```python
from build123d import *

# Parameters (mm, degrees)
BOSS_EXTRU_2_DEPTH   = 5
D_GAGEMENT_M21_D     = 2.4
D_GAGEMENT_M21_DEPTH = 10
D_GAGEMENT_M21_TIP   = 0.721032743
D_GAGEMENT_M81_D     = 8.2
D_GAGEMENT_M81_DEPTH = 10
D_GAGEMENT_M81_TIP   = 2.463528538
D_GAGEMENT_M22_D     = 2.4
D_GAGEMENT_M22_DEPTH = 10
D_GAGEMENT_M22_TIP   = 0.721032743
D_GAGEMENT_M82_D     = 8.2
D_GAGEMENT_M82_DEPTH = 10
D_GAGEMENT_M82_TIP   = 2.463528538
D_GAGEMENT_M31_D     = 3.4
D_GAGEMENT_M31_DEPTH = 5
D_GAGEMENT_M31_TIP   = 1.021463052


with BuildPart() as part:
    # Esquisse1 → Boss.-Extru.2 (new body)
    with BuildSketch(Plane.XY):
        with BuildLine():
            Line((-2.492714326, 26.224698366), (6.10421614, 33.170262072))
            ThreePointArc((6.10421614, 33.170262072), (7.000718602, 41.608051079), (-1.437070405, 42.504553542))
            Line((-1.437070405, 42.504553542), (-48.270643273, 4.667145735))
            ThreePointArc((-48.270643273, 4.667145735), (-50.15698128, -1.999640667), (-44.5, -6))
            Line((-44.5, -6), (44.5, -6))
            ThreePointArc((44.5, -6), (50.5, 0), (44.5, 6))
            Line((44.5, 6), (16.324378099, 6))
            Line((16.324378099, 6), (-2.492714326, 26.224698366))
        make_face()
        Polygon((-27.526006497, 6), (-0.066265486, 6), (-11.849799184, 18.664996768), align=None, mode=Mode.SUBTRACT)
        with BuildLine():
            ThreePointArc((-3.590453958, 35.622479779), (-3.889288112, 32.809883443), (-1.076691777, 32.511049289))
            Line((-1.076691777, 32.511049289), (3.590453958, 36.281692562))
            ThreePointArc((3.590453958, 36.281692562), (3.889288112, 39.094288898), (1.076691777, 39.393123052))
            Line((1.076691777, 39.393123052), (-3.590453958, 35.622479779))
        make_face(mode=Mode.SUBTRACT)
    extrude(amount=BOSS_EXTRU_2_DEPTH)

    # Dégagement M21
    with Locations(Plane(origin=(0, 0, 0), x_dir=(-1, 0, 0), z_dir=(0, 0, -1))):
        with Locations((44.5, 0), (30.5, 0)):
            Hole(D_GAGEMENT_M21_D / 2, depth=D_GAGEMENT_M21_DEPTH)
            with Locations((0, 0, -(D_GAGEMENT_M21_DEPTH + D_GAGEMENT_M21_TIP / 2))):  # 118° drill point
                Cone(0, D_GAGEMENT_M21_D / 2, D_GAGEMENT_M21_TIP, mode=Mode.SUBTRACT)

    # Dégagement M81
    with Locations(Plane(origin=(0, 0, 0), x_dir=(-1, 0, 0), z_dir=(0, 0, -1))):
        with Locations((37.5, 0)):
            Hole(D_GAGEMENT_M81_D / 2, depth=D_GAGEMENT_M81_DEPTH)
            with Locations((0, 0, -(D_GAGEMENT_M81_DEPTH + D_GAGEMENT_M81_TIP / 2))):  # 118° drill point
                Cone(0, D_GAGEMENT_M81_D / 2, D_GAGEMENT_M81_TIP, mode=Mode.SUBTRACT)

    # Dégagement M22
    with Locations(Plane(origin=(0, 0, 0), x_dir=(-1, 0, 0), z_dir=(0, 0, -1))):
        with Locations((-44.5, 0), (-30.5, 0)):
            Hole(D_GAGEMENT_M22_D / 2, depth=D_GAGEMENT_M22_DEPTH)
            with Locations((0, 0, -(D_GAGEMENT_M22_DEPTH + D_GAGEMENT_M22_TIP / 2))):  # 118° drill point
                Cone(0, D_GAGEMENT_M22_D / 2, D_GAGEMENT_M22_TIP, mode=Mode.SUBTRACT)

    # Dégagement M82
    with Locations(Plane.XY.offset(5)):
        with Locations((37.5, 0)):
            Hole(D_GAGEMENT_M82_D / 2, depth=D_GAGEMENT_M82_DEPTH)
            with Locations((0, 0, -(D_GAGEMENT_M82_DEPTH + D_GAGEMENT_M82_TIP / 2))):  # 118° drill point
                Cone(0, D_GAGEMENT_M82_D / 2, D_GAGEMENT_M82_TIP, mode=Mode.SUBTRACT)

    # Dégagement M31
    with Locations(Plane.XY.offset(5)):
        with Locations((-18.192282617, 21.254321849), (10.613248654, 0), (-10.613248654, 0)):
            Hole(D_GAGEMENT_M31_D / 2, depth=D_GAGEMENT_M31_DEPTH)
            with Locations((0, 0, -(D_GAGEMENT_M31_DEPTH + D_GAGEMENT_M31_TIP / 2))):  # 118° drill point
                Cone(0, D_GAGEMENT_M31_D / 2, D_GAGEMENT_M31_TIP, mode=Mode.SUBTRACT)


solid = part.part
```
Input: part model. Units: mm. Frame: model coordinates. A direction names the side the tool comes from. Give positions to 0.01 mm unless a question says otherwise; leave off trailing zeros. Order: outer loops, then holes, each group sorted by start corner. A loop starts at its lowest first (then second) coordinate and runs counter-clockwise, first axis right, second up. Notation, with made-up numbers: M 25,58 L 84,58 A14 ccw 84,76 Z; hole C 23.25,16.5 d5. An arc over 180 degrees is marked long. Return JSON: item names as keys, results as strings.
1) Line query: L1, parallel to Y at x = -17.5, z = 2.05; L2, parallel to Y at x = 30.5, z = 1.65; L3, parallel to Y at x = 34, z = 1.6. Output: solid intervals per line, ascending. Write a range as [from, to].
Taken from the geometry:
{"L1": "y = [-6, 6], [14.1, 19.7], [22.81, 29.53]", "L2": "y = [-6, -1.2], [1.2, 6]", "L3": "y = [-6, -2.14], [2.14, 6]"}
2) Section query A-A on x = 37.5. Output: boundary loops of the cut face in (y, z).
Taken from the geometry:
{"outline": "M -6,0 L -4.1,0 L -4.1,5 L -6,5 Z; M 4.1,0 L 6,0 L 6,5 L 4.1,5 Z"}
3) Contact query for flat-ended pins moving along their axis: pin 1 (3 mm diameter, centred on x = -18.19, y = 21.25, fed in from +Z); pin 2 (1.5 mm diameter, centred on y = 3.5, z = 4.5, fed in from +X); pin 3 (1.5 mm diameter, centred on x = 12.5, z = 3, fed in from +Y). Output: stop coordinate, or through.
Taken from the geometry:
{"pin 1": "passes through", "pin 2": "stops at x = 49.83", "pin 3": "stops at y = 10.92"}
4) Section query B-B on y = 0. Count the separate pieces of the cut face and the enclosed holes in it, and give its area (3 significant figures).
Taken from the geometry:
{"separate pieces": "9", "enclosed holes": "0", "area": "341 mm2"}
5) Access query for faces 4 (the face through (1.75, 29.65, 2.46)), 5 (the face through (-1, 8, 0)), 6 (the face through (-14, 6, 2)). Directions: +Z, -Z, +X, -X, +Y, -Y. A direction counts if a zero-diameter tool reaches every point of the face in a straight line with its end or side. Return the directions, or none.
Taken from the geometry:
{"face 4": "+Z, -Z, +X", "face 5": "-Z, +X, -X, +Y, -Y", "face 6": "+Z, -Z"}
6) Mould query, pull axis X, two halves, no side actions, for faces 1 (the face through (-1, 8, 5)), 2 (the face through (-1.224, 37.534, 2.465)), 3 (the face through (7.05, 15.97, 2.46)). Classes: released by +X, released by -X, zero draft, split by the parting line, or undercut.
Taken from the geometry:
{"face 1": "zero draft", "face 2": "undercut", "face 3": "released by +X"}
7) Section query D-D on y = 10. Output: boundary loops of the cut face in (x, z), and give its area (3 significant figures).
Taken from the geometry:
{"outline": "M -41.67,0 L -22.57,0 L -22.57,5 L -41.67,5 Z; M -3.79,0 L 12.6,0 L 12.6,5 L -3.79,5 Z", "area": "177 mm2"}
